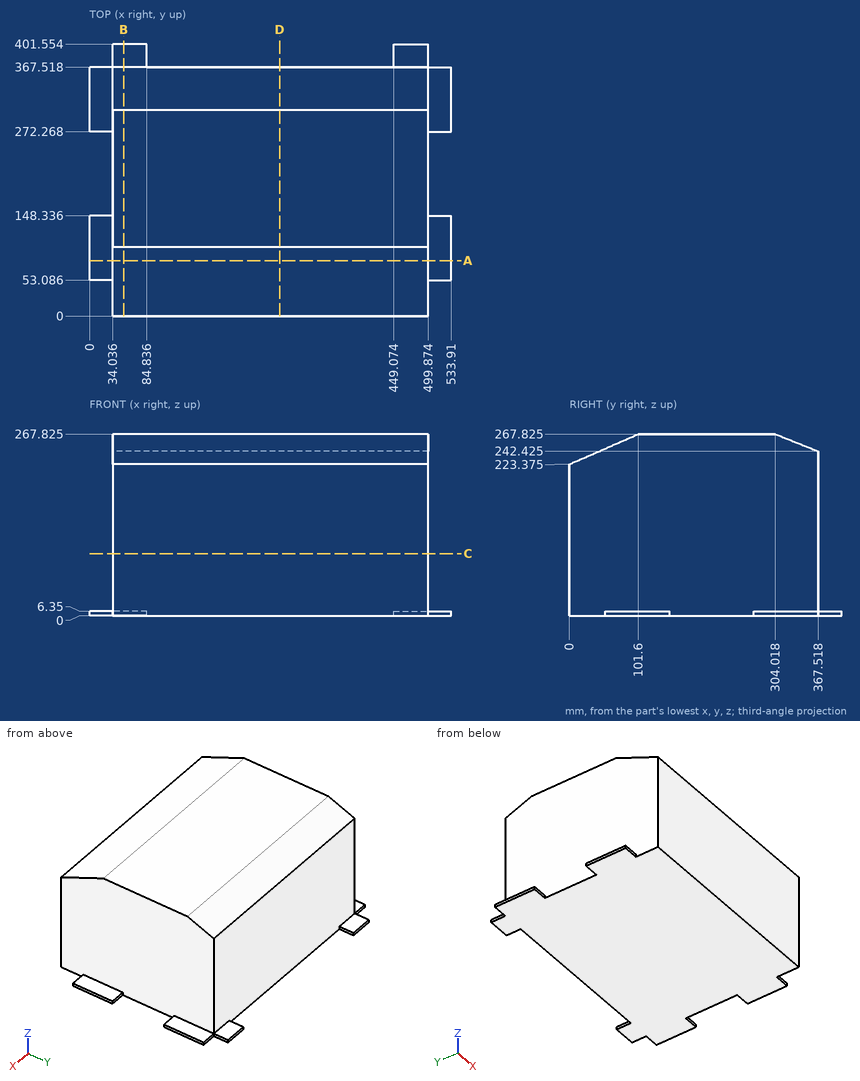
Job drawing, mm, ordinate dimensions from the low corner. One solid piece. Coordinates: 2 decimals unless noted, no trailing zeros. Loops run counter-clockwise (first coordinate to the right, second up) from the corner with the lowest first, then second, coordinate; pieces in that order, holes last. Notation, with made-up numbers: (64.5, -14.75) - (83.5, -14.75) arc R22 cw to (83.5, 15.25) - close; hole circle Ø7 at (50, 46). An arc over 180 degrees is marked (long way). Answer as a JSON object with one key per item and string values. Group by question number.
(1) Cut at D-D (x = 280.5). Give the cut face in (y, z) (3 decimals).
(2) Cut at C-C (z = 91.5). Give the cut face in (x, y).
(3) Cut at A-A (y = 82). Give the cut face in (x, z).
(4) Probe line 1 along Y through (x, z) = (75.5, 52.5); line 2 along X through (y, z) = (303, 99); line 3 along Z through (x, y) = (66, 50.5). List the from-to ranges inside material, lowest first.
(5) Flat gauge pins, fed straight in: pin 1 (5 mm diameter, centred on x = 21, z = 3.5, fed in from -Y); pin 2 (1.9 mm diameter, centred on y = 377.5, z = 2.5, fed in from -X); pin 3 (10 mm diameter, centred on x = 525, y = 93.5, fed in from +Z). Where does each tip first touch, or does it go through?
(6) Cut at B-B (x = 50.5). Give the cut face in (y, z) (3 decimals).
Geometry says:
{
 "1": {"outline": "(0, 0) - (367.518, 0) - (367.518, 242.425) - (304.018, 267.825) - (101.6, 267.825) - (0, 223.375) - close"},
 "2": {"outline": "(34.04, 0) - (499.87, 0) - (499.87, 367.52) - (34.04, 367.52) - close"},
 "3": {"outline": "(0, 0) - (533.91, 0) - (533.91, 6.35) - (499.87, 6.35) - (499.87, 259.25) - (34.04, 259.25) - (34.04, 6.35) - (0, 6.35) - close"},
 "4": {"line 1": "y = 0 to 367.52", "line 2": "x = 34.04 to 499.87", "line 3": "z = 0 to 245.47"},
 "5": {"pin 1": "stops at y = 53.09", "pin 2": "stops at x = 34.04", "pin 3": "stops at z = 6.35"},
 "6": {"outline": "(0, 0) - (401.554, 0) - (401.554, 6.35) - (367.518, 6.35) - (367.518, 242.425) - (304.018, 267.825) - (101.6, 267.825) - (0, 223.375) - close"}
}
